Build history of the part. All positions in model axes, mm. Face numbers are marked on the shaded views. A direction names the side the tool comes from. Round coordinates to 2 decimals unless told otherwise and drop trailing zeros. Write each loop counter-clockwise with the first axis right and the second up, starting at its lowest first coordinate (ties: lowest second). Pieces come first, ordered by that corner, then holes.
Item 1: Band-saw the part on A-A, the plane y = -0.7. Write the cut outline in (x, z).
Item 2: Drop flat-ended pins along their axis: pin 1 Ø3 at (y, z) = (1, -5) entering from +X; pin 2 Ø1.5 at (x, y) = (34, 1) entering from -Z. Give the stop position or say it passes through.
Item 3: Wall check: probe 1 along X at (y, z) = (-0.7, -14); probe 2 along Z at (x, y) = (32, -0.6). Give the ranges that are in metal, low to high.
Item 4: 3-axis set-ups, long thin cutter, end or side, ignore diameter. For the marked faces 1 and 2: which of +Z, -Z, +X, -X, +Y, -Y reach the whole face in a straight line?
Item 5: Band-saw the part on B-B, the plane z = -3. Write the cut outline in (x, y).
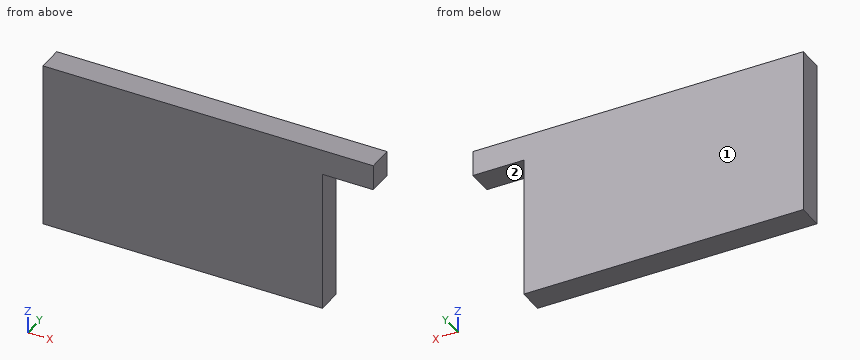
```python
from build123d import *

# Parameters (mm, degrees)
SKETCH1_W           = 55
SKETCH1_H           = 33
SKETCH1_W_2         = 10
SKETCH1_H_2         = 5
BOSS_EXTRUDE1_DEPTH = 2.5


with BuildPart() as part:
    # Sketch1 → Boss-Extrude1 (new body, symmetric)
    with BuildSketch(Plane(origin=(0, 0, 0), x_dir=(1, 0, 0), z_dir=(0, 1, 0))):
        Rectangle(SKETCH1_W, SKETCH1_H)
        with Locations((32.5, -14)):
            Rectangle(SKETCH1_W_2, SKETCH1_H_2)
    extrude(amount=BOSS_EXTRUDE1_DEPTH, both=True)


solid = part.part
```
Results:
1. outline: (-27.5, -16.5) - (27.5, -16.5) - (27.5, 11.5) - (37.5, 11.5) - (37.5, 16.5) - (-27.5, 16.5) - close
2. pin 1: stops at x = 27.5
2. pin 2: stops at z = 11.5
3. probe 1: x = -27.5 to 27.5
3. probe 2: z = 11.5 to 16.5
4. face 1: +Z, -Z, +X, -X, +Y
4. face 2: -Z, +X, +Y, -Y
5. outline: (-27.5, -2.5) - (27.5, -2.5) - (27.5, 2.5) - (-27.5, 2.5) - close
